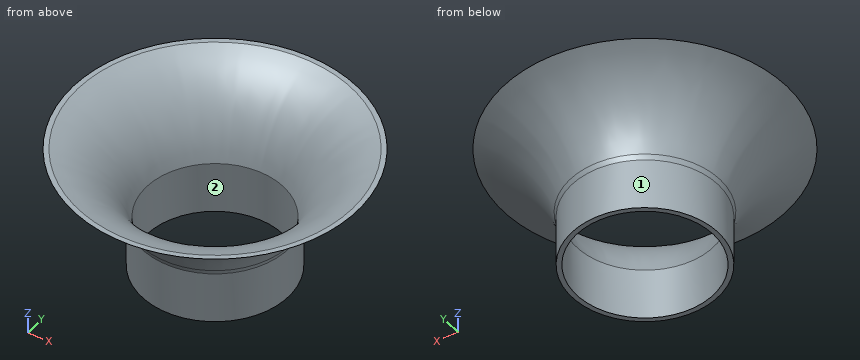
```python
from build123d import *


with BuildPart() as f1:
    # F0 (on Front) → F1 (revolve)
    with BuildSketch(Plane.XZ):
        with BuildLine():
            ThreePointArc((0, 0), (-5.096418, 9.276676), (-14, 15))
            Line((-14, 15), (-15, 15))
            ThreePointArc((-15, 15), (-6.581159, 9.540535), (-1.314101, 1))
            Line((-1.314101, 1), (-0.970255, 0))
            Line((-0.970255, 0), (-0.970255, -10.510325))
            Line((-0.970255, -10.510325), (0, -10.510325))
            Line((0, -10.510325), (0, 0))
        make_face()
    revolve(axis=Axis((14.029745, 0, 7.5), (0, 0, 1)))


solid = f1.part
```
Can you work these out from the model? Positions are in its coordinate system, mm. Face numbers are marked on the shaded views. Coordinates: 2 decimals unless noted, no trailing zeros. Loops run counter-clockwise (first coordinate to the right, second up) from the corner with the lowest first, then second, coordinate; pieces in that order, holes last.
1) Imagine slicing it at B-B on z = 6. List the corners of the cut face in (x, y) for me, plus the area to 3 significant figures.
2) Imagine slicing it at A-A on y = 0. List the corners of the cut face in (x, z) for me, plus the area to 3 significant figures.
3) Thinking about a two-plate mould opening in X: for the marked faces 1 and 2, which applies, pulls with the +X half, pulls with the -X half, needs draft (parallel to the pull), parting line crosses it, or undercut?
4) Imagine slicing it at C-C on z = -7.25. List the corners of the cut face in (x, y) for me, plus the area to 3 significant figures.
5) I need wall thicknesses on probe 1 along X at (y, z) = (0, -6.75); probe 2 along Y at (x, z) = (0.5, 14); probe 3 along Y at (x, z) = (8, -3.25). Which ranges of each line are inside material? Lowest first, please.
6) For pin 1 (5 mm diameter, centred on y = 2.5, z = 0, fed in from +X); pin 2 (2 mm diameter, centred on x = 16.5, y = 18.5, fed in from -Z); pin 3 (1.5 mm diameter, centred on x = -1.5, y = -11, fed in from -Z); pin 4 (2 mm diameter, centred on y = -20.5, z = 5, fed in from -X), each with a flat end and sliding along its axis, tell me the tip position at first contact or that it passes through.
Completed:
1. outline: circle Ø35.56 at (14.03, 0); hole circle Ø33.22 at (14.03, 0)
1. area: 126 mm2
2. outline: (-15, 15) arc R22.84 cw to (-1.31, 1) - (-0.97, 0) - (-0.97, -10.51) - (0, -10.51) - (0, 0) arc R21.51 ccw to (-14, 15) - close; (28.06, -10.51) - (29.03, -10.51) - (29.03, 0) - (29.37, 1) arc R22.84 cw to (43.06, 15) - (42.06, 15) arc R21.51 ccw to (28.06, 0) - close
2. area: 55.1 mm2
3. face 1: parting line crosses it
3. face 2: undercut
4. outline: circle Ø30 at (14.03, 0); hole circle Ø28.06 at (14.03, 0)
4. area: 88.5 mm2
5. probe 1: x = -0.97 to 0, 28.06 to 29.03
5. probe 2: y = -23.04 to -21.69, 21.69 to 23.04
5. probe 3: y = -13.73 to -12.67, 12.67 to 13.73
6. pin 1: stops at x = 29.8
6. pin 2: stops at z = 5.82
6. pin 3: stops at z = 6.74
6. pin 4: passes through
